Read the model definition and answer for the solid it produces. Units are mm, in the model's axes. A direction names the side the tool comes from. Coordinates: 2 decimals unless noted, no trailing zeros. Loops run counter-clockwise (first coordinate to the right, second up) from the corner with the lowest first, then second, coordinate; pieces in that order, holes last. Notation, with made-up numbers: (33, -34) -> (38, -34) arc R30 ccw to (38, -12) -> close; hole circle Ø11 at (37.5, -0.5). An arc over 180 degrees is marked (long way). Answer as a JSON object with one key per item and string values. Group by question number.
1) Which of the six approach directions +Z, -Z, +X, -X, +Y, -Y give full straight-line access (tool end or side, diameter ignored) to faces 1 (the face through (2.764, -1.528, 21.917)), 2 (the face through (-10, -2, -15)), 3 (the face through (-2.764, -1.528, -21.917)), 4 (the face through (10, -2, -15))?
2) Section A-A, the plane z = -10 is taken. Give the vertices of the cut face in (x, y), plus the area to 3 significant figures.
3) Section B-B, the plane x = 0 is taken. Give the vertices of the cut face in (y, z) (3 decimals).
4) Determine the mould class of faces 5 (the face through (8, -2, 18.875)), 6 (the face through (2.76, -1.53, -21.83)), 7 (the face through (6.308, -1.528, 20.379)), 8 (the face through (0.06, -1.53, 16.23)) for opening direction X: released by +X, released by -X, zero draft, split by the parting line, or undercut.
5) Consider probe 1 along Z at (x, y) = (0, -1.6) (3 decimals); probe 2 along X at (y, z) = (-0.35, -8); probe 3 along X at (y, z) = (-0.1, 22.5). Determine where each line is inside the solid, lowest interval first. Write a range as [from, to].
6) Section C-C, the plane y = -1.7 is taken. Count the separate pieces of the cut face and the enclosed holes in it, plus the area to 3 significant figures.
7) Section D-D, the plane z = 19.5 is taken. Give the vertices of the cut face in (x, y), plus the area to 3 significant figures.
8) Flat-ended cylindrical pins translate along their axes: P1, Ø8, axis at x = -3, z = 3, coming from the -Y side; P2, Ø1.6, axis at y = -2, z = 13.5, coming from the +X side; P3, Ø1, axis at x = -8, y = -1, coming from the +Z side (3 decimals); P4, Ø0.9, axis at y = -2, z = -13.5, coming from the -X side. Find the tip coordinate at first contact, or state that the pin passes through.
from build123d import *

# Parameters (mm, degrees)
F0_R     = 1.8
F0_R_2   = 6.375
F1_DEPTH = 3.1


with BuildPart() as f1:
    # F0 (on Front) → F1 (new body)
    with BuildSketch(Plane.XZ):
        with BuildLine():
            Line((-10, 18.875), (-10, 11.18034))
            ThreePointArc((-10, 11.18034), (-15, 0), (-10, -11.18034))
            Line((-10, -11.18034), (-10, -18.875))
            Line((-10, -18.875), (-6.25, -18.875))
            Line((-6.25, -18.875), (-6.367204, -21.925))
            Line((-6.367204, -21.925), (-6.525, -22.125))
            Line((-6.525, -22.125), (-6.152377, -24.536093))
            ThreePointArc((-6.152377, -24.536093), (-6.017418, -24.778675), (-5.75707, -24.875))
            Line((-5.75707, -24.875), (-2.877908, -24.875))
            Line((-2.877908, -24.875), (-2.647343, -18.875))
            ThreePointArc((-2.647343, -18.875), (0, -16.227657), (2.647343, -18.875))
            Line((2.647343, -18.875), (2.877908, -24.875))
            Line((2.877908, -24.875), (5.75707, -24.875))
            ThreePointArc((5.75707, -24.875), (6.017418, -24.778675), (6.152377, -24.536093))
            Line((6.152377, -24.536093), (6.525, -22.125))
            Line((6.525, -22.125), (6.367204, -21.925))
            Line((6.367204, -21.925), (6.25, -18.875))
            Line((6.25, -18.875), (10, -18.875))
            Line((10, -18.875), (10, -11.18034))
            ThreePointArc((10, -11.18034), (15, 0), (10, 11.18034))
            Line((10, 11.18034), (10, 18.875))
            Line((10, 18.875), (6.25, 18.875))
            Line((6.25, 18.875), (6.367204, 21.925))
            Line((6.367204, 21.925), (6.525, 22.125))
            Line((6.525, 22.125), (6.152377, 24.536093))
            ThreePointArc((6.152377, 24.536093), (6.017418, 24.778675), (5.75707, 24.875))
            Line((5.75707, 24.875), (2.877908, 24.875))
            Line((2.877908, 24.875), (2.647343, 18.875))
            ThreePointArc((2.647343, 18.875), (0, 16.227657), (-2.647343, 18.875))
            Line((-2.647343, 18.875), (-2.877908, 24.875))
            Line((-2.877908, 24.875), (-5.75707, 24.875))
            ThreePointArc((-5.75707, 24.875), (-6.017418, 24.778675), (-6.152377, 24.536093))
            Line((-6.152377, 24.536093), (-6.525, 22.125))
            Line((-6.525, 22.125), (-6.367204, 21.925))
            Line((-6.367204, 21.925), (-6.25, 18.875))
            Line((-6.25, 18.875), (-10, 18.875))
        make_face()
        with Locations((-7.071068, -7.071068)):
            Circle(F0_R, mode=Mode.SUBTRACT)
        with Locations((0, -10)):
            Circle(F0_R, mode=Mode.SUBTRACT)
        with Locations((7.071068, -7.071068)):
            Circle(F0_R, mode=Mode.SUBTRACT)
        with Locations((-10, 0)):
            Circle(F0_R, mode=Mode.SUBTRACT)
        with Locations((-7.071068, 7.071068)):
            Circle(F0_R, mode=Mode.SUBTRACT)
        Circle(F0_R_2, mode=Mode.SUBTRACT)
        with Locations((0, 10)):
            Circle(F0_R, mode=Mode.SUBTRACT)
        with Locations((7.071068, 7.071068)):
            Circle(F0_R, mode=Mode.SUBTRACT)
        with Locations((10, 0)):
            Circle(F0_R, mode=Mode.SUBTRACT)
    extrude(amount=F1_DEPTH)


solid = f1.part
Determined:
{
 "1": {"face 1": "+Z, +Y, -Y", "face 2": "-Z, -X, +Y, -Y", "face 3": "-Z, +Y, -Y", "face 4": "-Z, +X, +Y, -Y"},
 "2": {"outline": "(-11.18, -3.1) -> (-1.8, -3.1) -> (-1.8, 0) -> (-11.18, 0) -> close; (1.8, -3.1) -> (11.18, -3.1) -> (11.18, 0) -> (1.8, 0) -> close", "area": "58.2 mm²"},
 "3": {"outline": "(-3.1, -16.228) -> (0, -16.228) -> (0, -11.8) -> (-3.1, -11.8) -> close; (-3.1, -8.2) -> (0, -8.2) -> (0, -6.375) -> (-3.1, -6.375) -> close; (-3.1, 6.375) -> (0, 6.375) -> (0, 8.2) -> (-3.1, 8.2) -> close; (-3.1, 11.8) -> (0, 11.8) -> (0, 16.228) -> (-3.1, 16.228) -> close"},
 "4": {"face 5": "zero draft", "face 6": "undercut", "face 7": "released by +X", "face 8": "undercut"},
 "5": {"probe 1": "[-16.228, -11.8], [-8.2, -6.375], [6.375, 8.2], [11.8, 16.228]", "probe 2": "[-12.69, -8.61], [-5.53, 5.53], [8.61, 12.69]", "probe 3": "[-6.47, -2.79], [2.79, 6.47]"},
 "6": {"separate pieces": "1", "enclosed holes": "9", "area": "764 mm²"},
 "7": {"outline": "(-6.27, -3.1) -> (-2.67, -3.1) -> (-2.67, 0) -> (-6.27, 0) -> close; (2.67, -3.1) -> (6.27, -3.1) -> (6.27, 0) -> (2.67, 0) -> close", "area": "22.3 mm²"},
 "8": {"P1": "y = -3.1", "P2": "x = 10", "P3": "z = 18.875", "P4": "x = -10"}
}
